Geometry: final body of the model. Coordinates: model frame, mm. Face numbers are marked on the shaded views. A direction names the side the tool comes from. Round coordinates to 2 decimals unless told otherwise and drop trailing zeros. Loops run counter-clockwise (first coordinate to the right, second up) from the corner with the lowest first, then second, coordinate; pieces in that order, holes last. Notation, with made-up numbers: (87.5, -33) - (139.5, -33) arc R20 cw to (139.5, -23) - close; hole circle Ø1 at (41, 78.5). An arc over 180 degrees is marked (long way). Return JSON: item names as keys, results as strings. Group by question number.
1. First-contact query: pin 1 Ø1.5 at (x, y) = (27.5, 21.5) entering from +Z; pin 2 Ø1.5 at (x, y) = (44, -67) entering from +Z; pin 3 Ø3 at (y, z) = (-26, 11.5) entering from -X (3 decimals); pin 4 Ø12 at (y, z) = (-35.96, 26.13) entering from -X. Flat tips, straight axial feed; report the tip coordinate or a pass-through.
2. Section C-C on z = 0. Count the separate pieces of the cut face and the enclosed holes in it, and give its area (3 significant figures).
3. Set-up query: the marked faces 4 and 5. Return all of +Z, -Z, +X, -X, +Y, -Y with unobstructed straight access to the full face (end or side cutting, diameter ignored); none if empty.
4. Draft query along Y for the marked faces 1, 2 and 3. Return one class per face: +Y half, -Y half, draft (parallel to the pull), parting line (faces both ways), or undercut.
5. Section D-D on x = 32. Return loops of the section in (y, z).
6. Material intervals for probe 1 along Y at (x, z) = (35, 0); probe 2 along Z at (x, y) = (64, -12.5); probe 3 along Y at (x, z) = (19, 0), sorted ascending.
7. Section B-B on x = 59. Return loops of the section in (y, z).
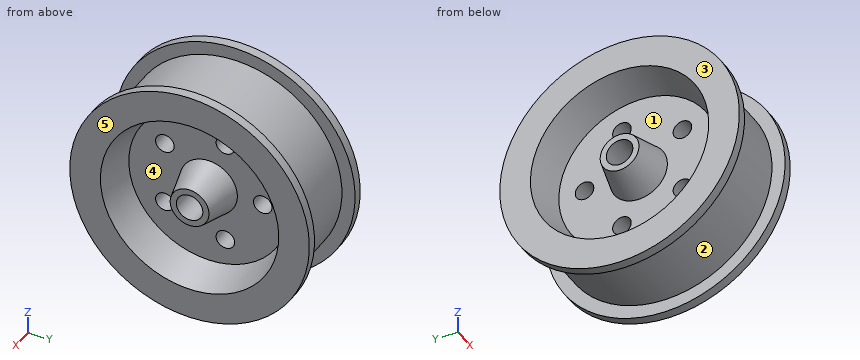
from build123d import *

# Parameters (mm, degrees)
ESBO_O2_R             = 7.62
CORTE_EXTRUS_O1_DEPTH = 162
PADR_OCIRCULAR1_COUNT = 5


with BuildPart() as part:
    # Esboço1 → Revolução1 (revolve)
    with BuildSketch(Plane.XY, mode=Mode.PRIVATE) as revolu_o1_sk:
        Polygon((0, 10.885714286), (76.2, 10.885714286), (76.2, 15.95320197), (47.625, 23.609850144), (47.625, 65.598953797), (76.2, 73.25560197), (76.2, 98.425), (68.504926108, 98.425), (68.504926108, 87.63), (7.695073892, 87.63), (7.695073892, 98.425), (0, 98.425), (0, 73.25560197), (28.575, 65.598953797), (28.575, 23.609850144), (0, 15.95320197), align=None)
    revolve(revolu_o1_sk.sketch.rotate(Axis((0, 0, 0), (1, 0, 0)), 90), axis=Axis((0, 0, 0), (1, 0, 0)))

    # Esboço2 → Corte-extrusão1 (cut)
    with BuildSketch(Plane.ZY.offset(-28.575)):
        with Locations((0, 44.45)):
            Circle(ESBO_O2_R)
    corte_extrus_o1 = extrude(amount=-CORTE_EXTRUS_O1_DEPTH, mode=Mode.SUBTRACT)

    # PadrãoCircular1: Corte-extrusão1 ×5 about axis
    padr_ocircular1_axis = Axis((0, 0, 0), (1, 0, 0))
    for i in range(1, PADR_OCIRCULAR1_COUNT):
        add(corte_extrus_o1.rotate(padr_ocircular1_axis, i * 360 / PADR_OCIRCULAR1_COUNT), mode=Mode.SUBTRACT)


solid = part.part
Taken from the geometry:
{
 "1": {"pin 1": "z = 85.14", "pin 2": "z = 57.36", "pin 3": "x = 28.575", "pin 4": "through"},
 "2": {"separate pieces": "3", "enclosed holes": "0", "area": "6,060 mm2"},
 "3": {"face 4": "+X", "face 5": "+Z, -Z, +X, +Y, -Y"},
 "4": {"face 1": "undercut", "face 2": "parting line", "face 3": "draft"},
 "5": {"outline": "circle Ø175.26 at (0, 0); hole circle Ø15.24 at (-35.96, -26.13); hole circle Ø15.24 at (-35.96, 26.13); hole circle Ø21.77 at (0, 0); hole circle Ø15.24 at (13.74, -42.27); hole circle Ø15.24 at (13.74, 42.27); hole circle Ø15.24 at (44.45, 0)"},
 "6": {"probe 1": "-87.63 to -10.89, 10.89 to 36.83, 52.07 to 87.63", "probe 2": "-86.73 to -68.86, -14.6 to 14.6, 68.86 to 86.73", "probe 3": "-87.63 to -68.16, -21.04 to -10.89, 10.89 to 21.04, 68.16 to 87.63"},
 "7": {"outline": "circle Ø175.26 at (0, 0); circle Ø41.12 at (0, 0); hole circle Ø137.29 at (0, 0); hole circle Ø21.77 at (0, 0)"}
}
